```python
from build123d import *

# Parameters (mm, degrees)
PAD_DEPTH       = 51
PAD001_DEPTH    = 53
PAD002_DEPTH    = 51
POCKET_DEPTH    = 51
POCKET001_DEPTH = 51
PAD003_DEPTH    = 39
PAD004_DEPTH    = 22
SKETCH009_W     = 5
SKETCH009_H     = 3
PAD005_DEPTH    = 51
SKETCH010_W     = 3
SKETCH010_H     = 2
POCKET002_DEPTH = 51
SKETCH011_W     = 5
SKETCH011_H     = 3
PAD006_DEPTH    = 51
SKETCH012_W     = 3
SKETCH012_H     = 2
POCKET003_DEPTH = 51
POCKET004_DEPTH = 140


with BuildPart() as part:
    # Sketch → Pad (new body)
    with BuildSketch(Plane.XY):
        Polygon((1, -3), (0, -2), (0, 0), (15, 0), (15, -2), (14, -3), align=None)
    extrude(amount=PAD_DEPTH)

    # Sketch001 (on Face4 of Pad) → Pad001 (join)
    with BuildSketch(Plane.YZ.offset(14)):
        Polygon((0, 33), (0, 18), (-2, 18), (-3, 19), (-3, 32), (-2, 33), align=None)
    extrude(amount=PAD001_DEPTH)

    # Sketch002 (on Face17 of Pad001) → Pad002 (join)
    with BuildSketch(Plane.XY):
        Polygon((66, 0), (81, 0), (81, -2), (80, -3), (67, -3), (66, -2), align=None)
    extrude(amount=PAD002_DEPTH)

    # Sketch003 (on Face5 of Pad002) → Pocket (cut)
    with BuildSketch(Plane.XY.offset(51)):
        Polygon((3, 0), (3, -1.5), (2.5, -1.5), (2.5, -2), (12.5, -2), (12.5, -1.5), (12, -1.5), (12, 0), align=None)
    extrude(amount=-POCKET_DEPTH, mode=Mode.SUBTRACT)

    # Sketch004 (on Face30 of Pocket) → Pocket001 (cut)
    with BuildSketch(Plane.XY.offset(51)):
        Polygon((78, 0), (69, 0), (69, -1.5), (68.5, -1.5), (68.5, -2), (78.5, -2), (78.5, -1.5), (78, -1.5), align=None)
    extrude(amount=-POCKET001_DEPTH, mode=Mode.SUBTRACT)

    # Sketch006 → Pad003 (join)
    with BuildSketch(Plane.YZ.offset(80)):
        Polygon((0, 33), (-2, 33), (-3, 32), (-3, 19), (-2, 18), (0, 18), align=None)
    extrude(amount=PAD003_DEPTH)

    # Sketch007 (on Face3 of Pad003) → Pad004 (join)
    with BuildSketch(Plane(origin=(1, 0, 0), x_dir=(0, -1, 0), z_dir=(-1, 0, 0))):
        Polygon((0, 33), (2, 33), (3, 32), (3, 19), (2, 18), (0, 18), align=None)
    extrude(amount=PAD004_DEPTH)

    # Sketch009 (on Face61 of Pad004) → Pad005 (join)
    with BuildSketch(Plane(origin=(0, 0, 51), x_dir=(1, 0, 0), z_dir=(0, 0, -1))):
        with Locations((116.5, 1.5)):
            Rectangle(SKETCH009_W, SKETCH009_H)
    extrude(amount=PAD005_DEPTH)

    # Sketch010 (on Face70 of Pad005) → Pocket002 (cut)
    with BuildSketch(Plane(origin=(0, 0, 0), x_dir=(1, 0, 0), z_dir=(0, 0, -1))):
        with Locations((117.5, 1)):
            Rectangle(SKETCH010_W, SKETCH010_H)
    extrude(amount=-POCKET002_DEPTH, mode=Mode.SUBTRACT)

    # Sketch011 (on Face17 of Pocket002) → Pad006 (join)
    with BuildSketch(Plane(origin=(0, 0, 51), x_dir=(1, 0, 0), z_dir=(0, 0, -1))):
        with Locations((-18.5, 1.5)):
            Rectangle(SKETCH011_W, SKETCH011_H)
    extrude(amount=PAD006_DEPTH)

    # Sketch012 (on Face32 of Pad006) → Pocket003 (cut)
    with BuildSketch(Plane(origin=(0, 0, 0), x_dir=(1, 0, 0), z_dir=(0, 0, -1))):
        with Locations((-19.5, 1)):
            Rectangle(SKETCH012_W, SKETCH012_H)
    extrude(amount=-POCKET003_DEPTH, mode=Mode.SUBTRACT)

    # Sketch008 (on Face51 of Pad004) → Pocket004 (cut)
    with BuildSketch(Plane.YZ.offset(119)):
        Polygon((0, 30), (-1.5, 30), (-1.5, 30.5), (-2, 30.5), (-2, 20.5), (-1.5, 20.5), (-1.5, 21), (0, 21), align=None)
    extrude(amount=-POCKET004_DEPTH, mode=Mode.SUBTRACT)


solid = part.part
```
The listing builds one solid part. Answer for the finished solid, in the listing's coordinates (mm). Give positions to 0.01 mm unless a question says otherwise; leave off trailing zeros. Loops run counter-clockwise (first coordinate to the right, second up) from the corner with the lowest first, then second, coordinate; pieces in that order, holes last. Notation, with made-up numbers: (57.5, 35.25) - (86.5, 35.25) arc R28 cw to (86.5, 69.25) - close; hole circle Ø11 at (38, 21). An arc over 180 degrees is marked (long way). Answer as CSV lines item,"result". Start each with the question number.
Item 1: A cutting plane is placed at A-A on x = 92.5. Determine the outline of the cut face in (y, z).
Item 2: A cutting plane is placed at B-B on y = -0.6. Count the separate pieces of the cut face and the enclosed holes in it, then the cut area to 3 significant figures.
Item 3: The mould has two halves that part along Y. Classify faces 1 (the face through (40.6, -1.5, 20.7)), 2 (the face through (40, 0, 19)), 3 (the face through (-16, -1, 42)): +Y half, -Y half, draft (parallel to the pull), parting line (faces both ways), or undercut.
Item 4: Find the intervals of material crossed by line 1 (X direction, y = -0.45, z = 47); line 2 (Z direction, x = 41.5, y = -1.05); line 3 (X direction, y = -1.55, z = 42), in increasing order. Write a range as from..to.
Item 5: Each of these flat-tipped pins is pushed along its axis until it touches: pin 1 (1 mm diameter, centred on y = -1, z = 12.5, fed in from -X); pin 2 (1.6 mm diameter, centred on x = -8, y = -0.5, fed in from +Z); pin 3 (0.8 mm diameter, centred on y = -1, z = 11, fed in from +X). Where does it stop, or does it pass through?
Item 6: A cutting plane is placed at D-D on x = 4.5. Determine the outline of the cut face in (y, z).
Found:
1,outline,"(-3, 19) - (-2, 18) - (0, 18) - (0, 21) - (-1.5, 21) - (-1.5, 20.5) - (-2, 20.5) - (-2, 30.5) - (-1.5, 30.5) - (-1.5, 30) - (0, 30) - (0, 33) - (-2, 33) - (-3, 32) - close"
2,separate pieces,"6"
2,enclosed holes,"0"
2,area,"1,270 mm^2"
3,face 1,"undercut"
3,face 2,"+Y half"
3,face 3,"draft"
4,line 1,"x = -18..-16, 0..3, 12..15, 66..69, 78..81, 114..116"
4,line 2,"z = 18..21, 30..33"
4,line 3,"x = -18..-16, 0..2.5, 12.5..15, 66..68.5, 78.5..81, 114..116"
5,pin 1,"stops at x = -18"
5,pin 2,"stops at z = 33"
5,pin 3,"stops at x = 116"
6,outline,"(-3, 0) - (-2, 0) - (-2, 51) - (-3, 51) - close"
